Here's how the part is built. I have some questions about the finished solid (model axes, mm). Face numbers are marked on the shaded views. A direction names the side the tool comes from. Give positions to 0.01 mm unless a question says otherwise; leave off trailing zeros. Write each loop counter-clockwise with the first axis right and the second up, starting at its lowest first coordinate (ties: lowest second). Pieces come first, ordered by that corner, then holes. Notation, with made-up numbers: M -32,-31 L 6,-31 A31 ccw 6,-6 Z; hole C 69,-33 d7. An arc over 180 degrees is marked long. Use one line per item in the form item = value. Start each with the question number.
from build123d import *

# Parameters (mm, degrees)
SKETCH1_R           = 2.5
BOSS_EXTRUDE1_DEPTH = 15


with BuildPart() as part:
    # Sketch1 → Boss-Extrude1 (new body)
    with BuildSketch(Plane(origin=(0, 0, 0), x_dir=(1, 0, 0), z_dir=(0, 1, 0))):
        with BuildLine():
            Line((-30, -35), (30, -35))
            Line((30, -35), (35, -35))
            ThreePointArc((35, -35), (40, -30), (35, -25))
            Line((35, -25), (33, -25))
            ThreePointArc((33, -25), (30.878679656, -24.121320344), (30, -22))
            Line((30, -22), (30, 22.098959323))
            ThreePointArc((30, 22.098959323), (30.878679656, 24.220279667), (33, 25.098959323))
            Line((33, 25.098959323), (35, 25.098959323))
            ThreePointArc((35, 25.098959323), (39.975198659, 30.596350827), (34.010151382, 35))
            Line((34.010151382, 35), (30, 35))
            Line((30, 35), (-30, 35))
            Line((-30, 35), (-35.989848618, 35))
            ThreePointArc((-35.989848618, 35), (-39.975198659, 29.601567819), (-35, 25.098959323))
            Line((-35, 25.098959323), (-33, 25.098959323))
            ThreePointArc((-33, 25.098959323), (-30.878679656, 24.220279667), (-30, 22.098959323))
            Line((-30, 22.098959323), (-30, -22))
            ThreePointArc((-30, -22), (-30.878679656, -24.121320344), (-33, -25))
            Line((-33, -25), (-35, -25))
            ThreePointArc((-35, -25), (-40, -30), (-35, -35))
            Line((-35, -35), (-30, -35))
        make_face()
        with Locations(Location((-35, 30.098959323, 0), (0, 0, 270))):
            Circle(SKETCH1_R, mode=Mode.SUBTRACT)
        with Locations(Location((35, 30.098959323, 0), (0, 0, 270))):
            Circle(SKETCH1_R, mode=Mode.SUBTRACT)
        with Locations(Location((35, -30, 0), (0, 0, 270))):
            Circle(SKETCH1_R, mode=Mode.SUBTRACT)
        with Locations(Location((-35, -30, 0), (0, 0, 270))):
            Circle(SKETCH1_R, mode=Mode.SUBTRACT)
    extrude(amount=BOSS_EXTRUDE1_DEPTH)


solid = part.part
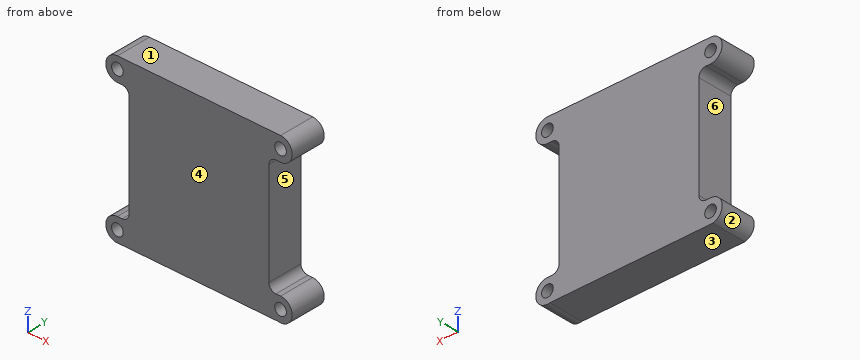
1) Thinking about a two-plate mould opening in Z: for the marked faces 1, 2 and 3, which applies, released by +Z, released by -Z, zero draft, split by the parting line, or undercut?
2) Suppose I cut it at A-A, the plane z = 30. List the corners of the cut face in (x, y) for me.
3) On a 3-axis mill with a long thin cutter (end or side, diameter ignored), from which of +Z, -Z, +X, -X, +Y, -Y can I reach the whole of each face in a straight line? I mean the marked faces 4, 5 and 6. Say none if no direction works.
4) Please list where these lines run through material, in increasing order: line 1 (X direction, y = 10.5, z = 30); line 2 (X direction, y = 5.25, z = 32); line 3 (Z direction, x = -36, y = 13).
5) Suppose I cut it at C-C, the plane z = 5.5. List the corners of the cut face in (x, y) for me, and give its area (3 significant figures).
6) Will these pins go through, and if not, where does the flat tip stop? P1, Ø4.5, axis at y = 6, z = 0, coming from the +X side; P2, Ø7.5, axis at x = -5, y = 4, coming from the -Z side; P3, Ø6, axis at y = 6.5, z = 7.5, coming from the -X side; P4, Ø6.5, axis at x = 35, z = -30.1, coming from the -Y side.
7) Suppose I cut it at B-B, the plane y = 8.75. List the corners of the cut face in (x, z) for me.
Checks:
q1.face_1 = released by +Z
q1.face_2 = undercut
q1.face_3 = released by -Z
q2.outline = M -40,0 L -37.5,0 L -37.5,15 L -40,15 Z; M -32.5,0 L 32.5,0 L 32.5,15 L -32.5,15 Z; M 37.5,0 L 40,0 L 40,15 L 37.5,15 Z
q3.face_4 = +Z, -Z, +X, -X, -Y
q3.face_5 = +X, +Y, -Y
q3.face_6 = -X, +Y, -Y
q4.line_1 = -40 to -37.5, -32.5 to 32.5, 37.5 to 40
q4.line_2 = -39.58 to -36.5, -33.5 to 33.5, 36.5 to 39.58
q4.line_3 = -35 to -32.39, -27.81 to -25.2, 25.1 to 27.71, 32.29 to 34.9
q5.outline = M -30,0 L 30,0 L 30,15 L -30,15 Z
q5.area = 900 mm^2
q6.P1 = 30
q6.P2 = -35
q6.P3 = -30
q6.P4 = 0
q7.outline = M -35.99,-35 L 34.01,-35 A5 ccw long 35,-25.1 L 33,-25.1 A3 cw 30,-22.1 L 30,22 A3 cw 33,25 L 35,25 A5 ccw 35,35 L -35,35 A5 ccw -35,25 L -33,25 A3 cw -30,22 L -30,-22.1 A3 cw -33,-25.1 L -35,-25.1 A5 ccw Z; hole C -35,-30.1 d5; hole C -35,30 d5; hole C 35,-30.1 d5; hole C 35,30 d5
